Source: three-view drawing plus pictorial views. Frame: mm from the lowest corner of the part. Give positions to 0.01 mm unless a question says otherwise; leave off trailing zeros. Write each loop counter-clockwise with the first axis right and the second up, starting at its lowest first coordinate (ties: lowest second). Pieces come first, ordered by that corner, then holes. Notation, with made-up numbers: (-5.5, 84.5) -> (48.5, 84.5) arc R18 cw to (48.5, 109.5) -> close; hole circle Ø10 at (7, -32.5). An arc over 180 degrees is marked (long way). Answer in a Markdown table with one row per item. Add a question column.
Item 1: Section query A-A on z = 6.5. Output: boundary loops of the cut face in (x, y).
Item 2: Section query B-B on y = 0.95. Output: boundary loops of the cut face in (x, z) (1 decimal).
Item 3: Section query C-C on z = 69. Output: boundary loops of the cut face in (x, y) (1 decimal).
Item 4: First-contact query: P1, Ø0.8, axis at y = 1, z = 70.5, coming from the -X side. Flat tip, straight axial feed; report the tip coordinate or a pass-through.
Item 5: Section query D-D on z = 80. Output: boundary loops of the cut face in (x, y).
Item 6: Material intervals for probe 1 along Z at (x, y) = (89.5, 0.6); probe 2 along X at (y, z) = (0.15, 52.5); probe 3 along Z at (x, y) = (79, 1.05) (1 decimal), sorted ascending. Write a range as from..to.
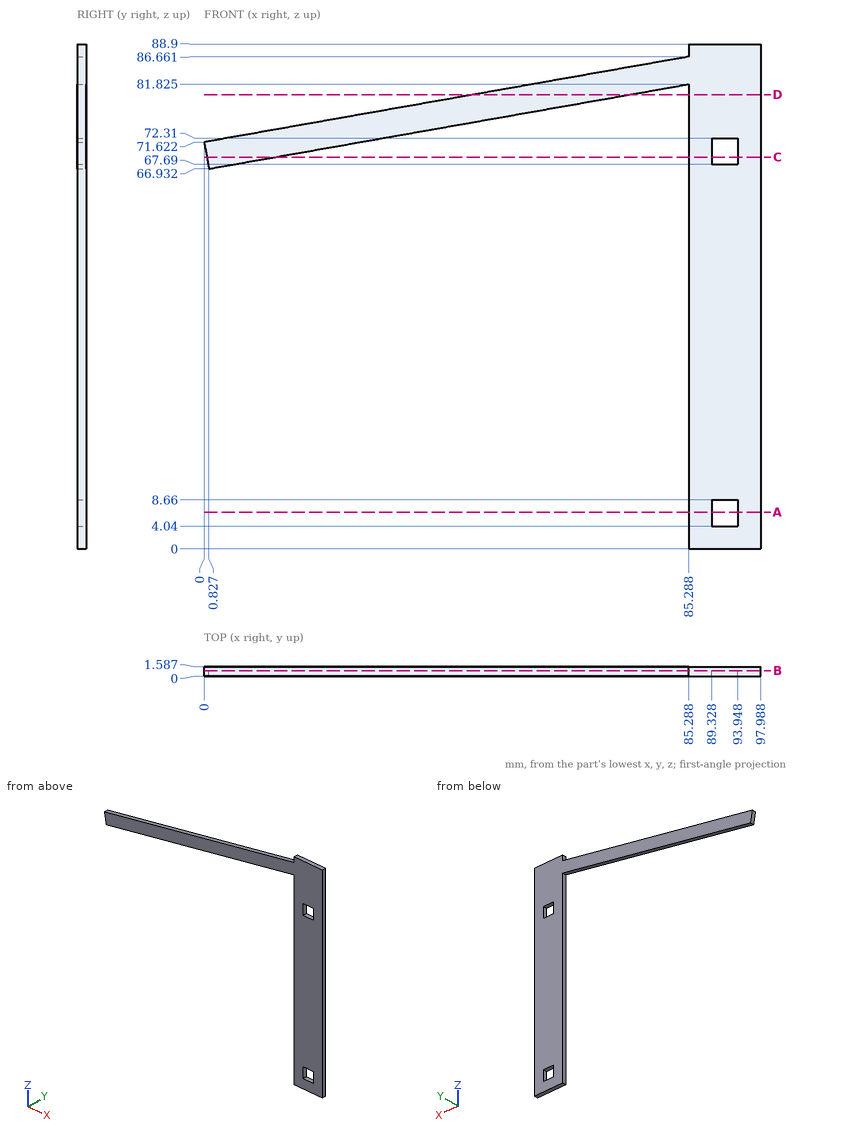
Findings below:
| question | item | result |
|---|---|---|
| 1 | outline | (85.29, 0) -> (89.33, 0) -> (89.33, 1.59) -> (85.29, 1.59) -> close; (93.95, 0) -> (97.99, 0) -> (97.99, 1.59) -> (93.95, 1.59) -> close |
| 2 | outline | (0, 71.6) -> (0.8, 66.9) -> (85.3, 81.8) -> (85.3, 0) -> (98, 0) -> (98, 88.9) -> (85.3, 88.9) -> (85.3, 86.7) -> close; hole (89.3, 4) -> (93.9, 4) -> (93.9, 8.7) -> (89.3, 8.7) -> close; hole (89.3, 67.7) -> (93.9, 67.7) -> (93.9, 72.3) -> (89.3, 72.3) -> close |
| 3 | outline | (0.5, 0) -> (12.6, 0) -> (12.6, 1.6) -> (0.5, 1.6) -> close; (85.3, 0) -> (89.3, 0) -> (89.3, 1.6) -> (85.3, 1.6) -> close; (93.9, 0) -> (98, 0) -> (98, 1.6) -> (93.9, 1.6) -> close |
| 4 | P1 | stops at x = 0.13 |
| 5 | outline | (47.51, 0) -> (74.94, 0) -> (74.94, 1.59) -> (47.51, 1.59) -> close; (85.29, 0) -> (97.99, 0) -> (97.99, 1.59) -> (85.29, 1.59) -> close |
| 6 | probe 1 | z = 0..4.04, 8.66..67.69, 72.31..88.9 |
| 6 | probe 2 | x = 85.29..97.99 |
| 6 | probe 3 | z = 80.7..85.6 |
